Part model, mm, in its own coordinate system. A direction names the side the tool comes from. Coordinates: 2 decimals unless noted, no trailing zeros. Order: outer loops, then holes, each group sorted by start corner. A loop starts at its lowest first (then second) coordinate and runs counter-clockwise, first axis right, second up. Notation, with made-up numbers: (-33.75, 84) - (-25.75, 84) arc R26 cw to (-25.75, 120) - close; hole circle Ø7 at (-26.5, -34.5). An arc over 180 degrees is marked (long way). Use a Markdown table: item, result. Add a question column.
1) Saw through at B-B on x = 0. List the corners of the cut face in (y, z), then the cut area to 3 significant figures.
2) Saw through at D-D on y = -21. List the corners of the cut face in (x, z), then the cut area to 3 significant figures.
3) Saw through at C-C on z = 4. List the corners of the cut face in (x, y), then the cut area to 3 significant figures.
4) Tool access for faces 1 (the face through (-11.5, -18.6, 4.07)), 2 (the face through (0, 14, 4)): list every direction of +Z, -Z, +X, -X, +Y, -Y with a clear straight run to the whole face (end or side of a thin tool).
5) Drop flat-ended pins along their axis: P1, Ø4, axis at x = 10, z = 5.5, coming from the +Y side; P2, Ø1.8, axis at x = -10, z = 4, coming from the -Y side. Give the stop position or say it passes through.
6) Wall check: L1, parallel to Y at x = 0, z = 6.5; L2, parallel to Z at x = -10, y = -20.5; L3, parallel to X at y = -22.5, z = 5. Give the ranges that are in metal, low to high. Write a range as [from, to].
7) Saw through at A-A on y = -10.5. List the corners of the cut face in (x, z).
8) Two-plate mould, pull along Y, no slides. Class faces 3 (the face through (5.97, 9.36, 3.94)), 4 (the face through (-10, -11, 4)), 5 (the face through (14, -13, 4)): +Y half, -Y half, draft (parallel to the pull), parting line (faces both ways), or undercut.
```python
from build123d import *

# Parameters (mm, degrees)
ESQUISSE1_R             = 11.1
BOSS_EXTRU_1_DEPTH      = 8
ESQUISSE2_R             = 1.5
ENL_V_MAT_EXTRU_1_DEPTH = 15


with BuildPart() as part:
    # Esquisse1 → Boss.-Extru.1 (new body)
    with BuildSketch(Plane.XY):
        with BuildLine():
            Line((-14, 0), (-14, -26))
            Line((-14, -26), (14, -26))
            Line((14, -26), (14, 0))
            ThreePointArc((14, 0), (0, 14), (-14, 0))
        make_face()
        Circle(ESQUISSE1_R, mode=Mode.SUBTRACT)
    extrude(amount=BOSS_EXTRU_1_DEPTH)

    # Esquisse2 → Enlèv. mat.-Extru.1 (cut)
    with BuildSketch(Plane.XZ.offset(26)):
        with Locations((-10, 4)):
            Circle(ESQUISSE2_R)
        with Locations((10, 4)):
            Circle(ESQUISSE2_R)
    extrude(amount=-ENL_V_MAT_EXTRU_1_DEPTH, mode=Mode.SUBTRACT)


solid = part.part
```
Results are:
| question | item | result |
|---|---|---|
| 1 | outline | (-26, 0) - (-11.1, 0) - (-11.1, 8) - (-26, 8) - close; (11.1, 0) - (14, 0) - (14, 8) - (11.1, 8) - close |
| 1 | area | 142 mm2 |
| 2 | outline | (-14, 0) - (14, 0) - (14, 8) - (-14, 8) - close; hole circle Ø3 at (-10, 4); hole circle Ø3 at (10, 4) |
| 2 | area | 210 mm2 |
| 3 | outline | (-14, -26) - (-11.5, -26) - (-11.5, -11) - (-8.5, -11) - (-8.5, -26) - (8.5, -26) - (8.5, -11) - (11.5, -11) - (11.5, -26) - (14, -26) - (14, 0) arc R14 ccw to (-14, 0) - close; hole circle Ø22.2 at (0, 0) |
| 3 | area | 559 mm2 |
| 4 | face 1 | -Y |
| 4 | face 2 | +Z, -Z, +Y |
| 5 | P1 | y = 11.49 |
| 5 | P2 | y = -11 |
| 6 | L1 | [-26, -11.1], [11.1, 14] |
| 6 | L2 | [0, 2.5], [5.5, 8] |
| 6 | L3 | [-14, -11.12], [-8.88, 8.88], [11.12, 14] |
| 7 | outline | (-14, 0) - (-3.6, 0) - (-3.6, 8) - (-14, 8) - close; (3.6, 0) - (14, 0) - (14, 8) - (3.6, 8) - close |
| 8 | face 3 | undercut |
| 8 | face 4 | -Y half |
| 8 | face 5 | draft |
